Verification items for the finished model (mm, model axes). A direction names the side the tool comes from. Round coordinates to 2 decimals unless told otherwise and drop trailing zeros. Write each loop counter-clockwise with the first axis right and the second up, starting at its lowest first coordinate (ties: lowest second). Pieces come first, ordered by that corner, then holes. Notation, with made-up numbers: M 12,13.25 L 66,13.25 A23 ccw 66,23.25 Z; hole C 23,89.25 d6. An arc over 180 degrees is marked long. One line per item, written item: value. Start each with the question number.
Item 1: Thickness scan on probe 1 along X at (y, z) = (16, 0); probe 2 along X at (y, z) = (5, 0); probe 3 along Z at (x, y) = (1, 10.5). Record the ranges inside material, lowest first. Write a range as from..to.
Item 2: Section check A-A, the plane x = 0. Record the cut outline in (y, z).
Item 3: Section check D-D, the plane z = -29. Record the cut outline in (x, y), then the cut area to 3 significant figures.
Item 4: Tool access check on faces 1 (the face through (1, 0, 26)), 2 (the face through (-39, 25, 12)), 3 (the face through (-39.05, 17.11, -8.67)). Record the directions out of +Z, -Z, +X, -X, +Y, -Y that give a thin tool (end or side, any length) a straight path to the whole face; none if there is none.
Item 5: Gauge pin test, flat ends, axial feed: pin 1 (8 mm diameter, centred on y = 1.5, z = -28, fed in from +X); pin 2 (4 mm diameter, centred on y = 6, z = -32, fed in from +X); pin 3 (6.5 mm diameter, centred on x = 0, z = 0, fed in from +Y); pin 4 (3 mm diameter, centred on x = -6, z = 43.5, fed in from -Y). Record the tip position at first contact, or that the pin passes through.
Item 6: Section check B-B, the plane z = 0. Record the cut outline in (x, y).
Item 7: Section check C-C, the plane y = 19. Record the cut outline in (x, z).
Item 8: Draft check along X on faces 4 (the face through (-0.3, -16, 4.2)), 5 (the face through (19.524, -7.888, -4.336)), 6 (the face through (-3.905, 4.213, 0.867)). Enter one of: +X half, -X half, draft (parallel to the pull), parting line (faces both ways), or undercut.
from build123d import *

# Parameters (mm, degrees)
SKETCH1_R           = 60
BOSS_EXTRUDE1_DEPTH = 25
SKETCH2_R           = 40
SKETCH2_R_2         = 20
CUT_EXTRUDE1_DEPTH  = 16
SKETCH3_R           = 20
BOSS_EXTRUDE2_DEPTH = 16
SKETCH4_R           = 4
CUT_EXTRUDE2_DEPTH  = 41


with BuildPart() as part:
    # Sketch1 → Boss-Extrude1 (new body)
    with BuildSketch(Plane(origin=(0, 0, 0), x_dir=(1, 0, 0), z_dir=(0, 1, 0))):
        with Locations(Location((0, 0, 0), (0, 0, 270))):
            Circle(SKETCH1_R)
    extrude(amount=BOSS_EXTRUDE1_DEPTH)

    # Sketch2 → Cut-Extrude1 (cut)
    with BuildSketch(Plane(origin=(0, 25, 0), x_dir=(1, 0, 0), z_dir=(0, 1, 0))):
        with Locations(Location((0, 0, 0), (0, 0, 270))):
            Circle(SKETCH2_R)
        with Locations(Location((0, 0, 0), (0, 0, 270))):
            Circle(SKETCH2_R_2, mode=Mode.SUBTRACT)
    extrude(amount=-CUT_EXTRUDE1_DEPTH, mode=Mode.SUBTRACT)

    # Sketch3 → Boss-Extrude2 (add)
    with BuildSketch(Plane.XZ):
        with Locations(Location((0, 0, 0), (0, 0, 90))):
            Circle(SKETCH3_R)
    extrude(amount=BOSS_EXTRUDE2_DEPTH)

    # Sketch4 → Cut-Extrude2 (cut)
    with BuildSketch(Plane.XZ.offset(16)):
        with Locations(Location((0, 0, 0), (0, 0, 270))):
            Circle(SKETCH4_R)
    extrude(amount=-CUT_EXTRUDE2_DEPTH, mode=Mode.SUBTRACT)


solid = part.part
Response values:
1. probe 1: x = -60..-40, -20..-4, 4..20, 40..60
1. probe 2: x = -60..-4, 4..60
1. probe 3: z = -59.99..-39.99, -19.97..-3.87, 3.87..19.97, 39.99..59.99
2. outline: M -16,-20 L 0,-20 L 0,-60 L 25,-60 L 25,-40 L 9,-40 L 9,-20 L 25,-20 L 25,-4 L -16,-4 Z; M -16,4 L 25,4 L 25,20 L 9,20 L 9,40 L 25,40 L 25,60 L 0,60 L 0,20 L -16,20 Z
3. outline: M -52.53,0 L 52.53,0 L 52.53,25 L 27.55,25 L 27.55,9 L -27.55,9 L -27.55,25 L -52.53,25 Z
3. area: 1,740 mm2
4. face 1: -Y
4. face 2: +Z, -Z, +X, -X, +Y
4. face 3: +Y
5. pin 1: stops at x = 54.99
5. pin 2: stops at x = 51.96
5. pin 3: passes through
5. pin 4: stops at y = 0
6. outline: M -60,0 L -20,0 L -20,-16 L -4,-16 L -4,25 L -20,25 L -20,9 L -40,9 L -40,25 L -60,25 Z; M 4,-16 L 20,-16 L 20,0 L 60,0 L 60,25 L 40,25 L 40,9 L 20,9 L 20,25 L 4,25 Z
7. outline: C 0,0 d120; C 0,0 d40; hole C 0,0 d80; hole C 0,0 d8
8. face 4: draft
8. face 5: parting line
8. face 6: undercut
